Geometry check sheet. Reference: the model listing, model coordinates, mm. A direction names the side the tool comes from. Round coordinates to 2 decimals unless told otherwise and drop trailing zeros. Loops run counter-clockwise (first coordinate to the right, second up) from the corner with the lowest first, then second, coordinate; pieces in that order, holes last.
```python
from build123d import *

# Parameters (mm, degrees)
SKETCH1_W                   = 9
SKETCH1_H                   = 6
MAIN_BODY_EXT_DEPTH         = 8.3
EMISSION_PATH_EXT_DEPTH     = 9
SKETCH3_R                   = 1.25
EMISSION_AND_GRIN_CUT_DEPTH = 19.125672401
SKETCH4_R                   = 1
DRUM_LENS_CUT_DEPTH         = 7
SKETCH5_W                   = 9
SKETCH5_H                   = 7.3
FILTERSET_CUT1_DEPTH        = 1
FILTERSET_CUT2_DEPTH        = 4
SKETCH10_R                  = 2.5
EMISSION_LENS_CUT_DEPTH     = 8.5
SKETCH15_R                  = 0.795
MAGNETS_CUT_DEPTH           = 0.9
SCREW_HOLES_CUT_DEPTH       = 19.561788707
SCREW_HOLES_CUT_DEPTH_BACK  = 3
SKETCH18_R                  = 0.375
EXTERNAL_FILLET_1_R         = 1.5
CUT_EXTRUDE8_DEPTH          = 12.545128843
CUT_EXTRUDE8_DEPTH_BACK     = 4
SKETCH28_R                  = 1.5
CUT_EXTRUDE9_DEPTH          = 3
CUT_EXTRUDE10_DEPTH         = 0.7
SKETCH29_R                  = 0.375
CUT_EXTRUDE11_DEPTH         = 2.5
SKETCH32_W                  = 2
SKETCH32_H                  = 2.36
CUT_EXTRUDE14_DEPTH         = 0.7
CUT_EXTRUDE16_DEPTH         = 9
CUT_EXTRUDE17_REACH         = 12.329
SKETCH37_R                  = 2
CUT_EXTRUDE18_START         = -9
CUT_EXTRUDE18_DEPTH         = 9


with BuildPart() as part:
    # Sketch1 → Main Body Ext (new body)
    with BuildSketch(Plane(origin=(0, 0, 0), x_dir=(1, 0, 0), z_dir=(0, 1, 0))):
        Rectangle(SKETCH1_W, SKETCH1_H)
    extrude(amount=MAIN_BODY_EXT_DEPTH)

    # Sketch8 → Emission Path Ext (add)
    with BuildSketch(Plane(origin=(0, 8.3, 0), x_dir=(1, 0, 0), z_dir=(0, 1, 0))):
        Polygon((0.25, 3), (1.5, 1.75), (1.5, -3), (-4.5, -3), (-4.5, 3), align=None)
    extrude(amount=EMISSION_PATH_EXT_DEPTH)

    # Sketch3 → Emission and Grin Cut (cut, through all)
    with BuildSketch(Plane.XZ):
        with Locations(Location((-1.5, 0, 0), (0, 0, 270))):
            Circle(SKETCH3_R)
    extrude(amount=-EMISSION_AND_GRIN_CUT_DEPTH, mode=Mode.SUBTRACT)

    # Sketch4 → Drum Lens Cut (cut)
    with BuildSketch(Plane(origin=(4.5, 0, 0), x_dir=(0, 0, -1), z_dir=(1, 0, 0))):
        with Locations((0, 3)):
            Circle(SKETCH4_R)
    extrude(amount=-DRUM_LENS_CUT_DEPTH, mode=Mode.SUBTRACT)

    # Sketch5 → FilterSet Cut1 (cut)
    with BuildSketch(Plane.XY.offset(3)):
        with Locations((0, 4.65)):
            Rectangle(SKETCH5_W, SKETCH5_H)
    extrude(amount=-FILTERSET_CUT1_DEPTH, mode=Mode.SUBTRACT)

    # Sketch6 → FilterSet Cut2 (cut)
    with BuildSketch(Plane.XY.offset(2)):
        with BuildLine():
            Line((2.3, 4.5), (2.3, 1.8))
            ThreePointArc((2.3, 1.8), (2.7, 1.4), (2.3, 1))
            Line((2.3, 1), (1.1, 1))
            ThreePointArc((1.1, 1), (0.7, 1.4), (1.1, 1.8))
            Line((1.1, 1.8), (1.1, 4.5))
            ThreePointArc((1.1, 4.5), (1.7, 5.1), (2.3, 4.5))
        make_face()
        with BuildLine():
            Line((-3.9, 7.9), (-3.9, 7.5))
            ThreePointArc((-3.9, 7.5), (-3.782842712, 7.217157288), (-3.5, 7.1))
            Line((-3.5, 7.1), (0.5, 7.1))
            ThreePointArc((0.5, 7.1), (0.782842712, 7.217157288), (0.9, 7.5))
            Line((0.9, 7.5), (0.9, 7.9))
            ThreePointArc((0.9, 7.9), (0.782842712, 8.182842712), (0.5, 8.3))
            Line((0.5, 8.3), (-3.5, 8.3))
            ThreePointArc((-3.5, 8.3), (-3.782842712, 8.182842712), (-3.9, 7.9))
        make_face()
        with BuildLine():
            Line((0.39411255, 6.591168825), (-3.848528137, 2.348528137))
            ThreePointArc((-3.848528137, 2.348528137), (-3.848528137, 1.5), (-3, 1.5))
            Line((-3, 1.5), (1.242640687, 5.742640687))
            ThreePointArc((1.242640687, 5.742640687), (1.242640687, 6.591168825), (0.39411255, 6.591168825))
        make_face()
    extrude(amount=-FILTERSET_CUT2_DEPTH, mode=Mode.SUBTRACT)

    # Sketch10 → Emission Lens Cut (cut)
    with BuildSketch(Plane(origin=(0, 17.3, 0), x_dir=(1, 0, 0), z_dir=(0, 1, 0))):
        with Locations(Location((-1.5, 0, 0), (0, 0, 270))):
            Circle(SKETCH10_R)
    extrude(amount=-EMISSION_LENS_CUT_DEPTH, mode=Mode.SUBTRACT)

    # Sketch15 → Magnets Cut (cut)
    with BuildSketch(Plane.XZ):
        with Locations(Location((-3.25, -1.875, 0), (0, 0, 270))):
            Circle(SKETCH15_R)
        with Locations(Location((-3.25, 1.875, 0), (0, 0, 270))):
            Circle(SKETCH15_R)
        with Locations(Location((1.5, 0, 0), (0, 0, 270))):
            Circle(SKETCH15_R)
    extrude(amount=-MAGNETS_CUT_DEPTH, mode=Mode.SUBTRACT)

    # Sketch18 → Screw Holes Cut (cut, two sides: drawn at the far end of the back side and taken through both)
    with BuildSketch(Plane.XY.offset(2).offset(-SCREW_HOLES_CUT_DEPTH_BACK)):
        with Locations(Location((-3.5, 4, 0), (0, 0, 180))):
            Circle(SKETCH18_R)
        with Locations(Location((2.5, 6.5, 0), (0, 0, 180))):
            Circle(SKETCH18_R)
        with Locations((3.25, 1)):
            Circle(SKETCH18_R)
    extrude(amount=SCREW_HOLES_CUT_DEPTH + SCREW_HOLES_CUT_DEPTH_BACK, mode=Mode.SUBTRACT)

    # External Fillet 1
    # the kernel refuses this fillet: 1.5 mm, written as the material it takes off along each edge
    with BuildSketch(Plane(origin=(-4.5, -3.75, -3), x_dir=(1, 0, 0), z_dir=(0, 1, 0))) as external_fillet_1_piece_1:
        with BuildLine():
            CenterArc((EXTERNAL_FILLET_1_R, -EXTERNAL_FILLET_1_R), EXTERNAL_FILLET_1_R, 90, 90)
            Line((0, -EXTERNAL_FILLET_1_R), (0, 0))
            Line((0, 0), (EXTERNAL_FILLET_1_R, 0))
        make_face()
    extrude(amount=24.8, mode=Mode.SUBTRACT)
    with BuildSketch(Plane(origin=(1.5, 8.3, 3), x_dir=(0, 0, -1), z_dir=(0, 1, 0))) as external_fillet_1_piece_2:
        with BuildLine():
            CenterArc((EXTERNAL_FILLET_1_R, EXTERNAL_FILLET_1_R), EXTERNAL_FILLET_1_R, 180, 90)
            Line((0, EXTERNAL_FILLET_1_R), (0, 0))
            Line((0, 0), (EXTERNAL_FILLET_1_R, 0))
        make_face()
    extrude(amount=12.75, mode=Mode.SUBTRACT)

    # Sketch28 → Cut-Extrude8 (cut, two sides: drawn at the far end of the back side and taken through both)
    with BuildSketch(Plane(origin=(0, 7.1, 0), x_dir=(1, 0, 0), z_dir=(0, 1, 0)).offset(-CUT_EXTRUDE8_DEPTH_BACK)):
        with Locations(Location((-1.5, 0, 0), (0, 0, 180))):
            Circle(SKETCH28_R)
    extrude(amount=CUT_EXTRUDE8_DEPTH + CUT_EXTRUDE8_DEPTH_BACK, mode=Mode.SUBTRACT)

    # Sketch14 → Cut-Extrude9 (cut)
    with BuildSketch(Plane.XZ):
        Polygon((4.5, -3), (4.5, -2.006698359), (3.837798906, -3), align=None)
    extrude(amount=-CUT_EXTRUDE9_DEPTH, mode=Mode.SUBTRACT)

    # Sketch12 → Cut-Extrude10 (cut)
    with BuildSketch(Plane(origin=(4.5, 0, 0), x_dir=(0, 0, -1), z_dir=(1, 0, 0))):
        with BuildLine():
            Line((1.6, 5.94), (-1.6, 5.94))
            Line((-1.6, 5.94), (-2, 5.94))
            Line((-2, 5.94), (-2, 1.33))
            Line((-2, 1.33), (1.6, 1.33))
            ThreePointArc((1.6, 1.33), (1.882842712, 1.447157288), (2, 1.73))
            Line((2, 1.73), (2, 5.54))
            ThreePointArc((2, 5.54), (1.882842712, 5.822842712), (1.6, 5.94))
        make_face()
    extrude(amount=-CUT_EXTRUDE10_DEPTH, mode=Mode.SUBTRACT)

    # Sketch29 → Cut-Extrude11 (cut)
    with BuildSketch(Plane(origin=(4.5, 0, 0), x_dir=(0, 0, -1), z_dir=(1, 0, 0))):
        with Locations((2, 6.5)):
            Circle(SKETCH29_R)
    extrude(amount=-CUT_EXTRUDE11_DEPTH, mode=Mode.SUBTRACT)

    # Sketch32 → Cut-Extrude14 (cut)
    with BuildSketch(Plane(origin=(4.5, 0, 0), x_dir=(0, 0, -1), z_dir=(1, 0, 0))):
        with Locations((0, 7.12)):
            Rectangle(SKETCH32_W, SKETCH32_H)
    extrude(amount=-CUT_EXTRUDE14_DEPTH, mode=Mode.SUBTRACT)

    # Sketch33 → Cut-Revolve1 (revolve, cut)
    with BuildSketch(Plane.XY, mode=Mode.PRIVATE) as cut_revolve1_sk:
        with BuildLine():
            Line((3.8, 3), (2.3, 3))
            ThreePointArc((2.3, 3), (2.739339828, 4.060660172), (3.8, 4.5))
            Line((3.8, 4.5), (3.8, 3))
        make_face()
    revolve(cut_revolve1_sk.sketch.rotate(Axis((3.8, 3, 0), (-1, 0, 0)), 90), axis=Axis((3.8, 3, 0), (-1, 0, 0)), mode=Mode.SUBTRACT)

    # Sketch36 → Cut-Extrude16 (cut)
    with BuildSketch(Plane(origin=(0, 17.3, 0), x_dir=(1, 0, 0), z_dir=(0, 1, 0))):
        with BuildLine():
            Line((-4.5, -1.5), (-4.5, -3))
            Line((-4.5, -3), (-3, -3))
            ThreePointArc((-3, -3), (-4.060660172, -2.560660172), (-4.5, -1.5))
        make_face()
    extrude(amount=-CUT_EXTRUDE16_DEPTH, mode=Mode.SUBTRACT)

    # Sketch37 → Cut-Extrude17 (cut, up to next)
    with BuildSketch(Plane(origin=(0, 8.8, 0), x_dir=(1, 0, 0), z_dir=(0, 1, 0)), mode=Mode.PRIVATE) as cut_extrude17_sk1:
        with Locations(Location((-1.5, 0, 0), (0, 0, 180))):
            Circle(SKETCH37_R)
    cut_extrude17_tool1 = extrude(cut_extrude17_sk1.sketch, amount=-CUT_EXTRUDE17_REACH, mode=Mode.PRIVATE) & part.part
    add(cut_extrude17_tool1.solids().sort_by_distance((-1.5, 8.8, 0))[0], mode=Mode.SUBTRACT)

    # Sketch38 → Cut-Extrude18 (cut)
    with BuildSketch(Plane(origin=(0, 17.3, 0), x_dir=(1, 0, 0), z_dir=(0, 1, 0)).offset(CUT_EXTRUDE18_START)):
        with BuildLine():
            Line((-3, 3), (0.25, 3))
            Line((0.25, 3), (1.5, 1.75))
            Line((1.5, 1.75), (1.5, -1.5))
            ThreePointArc((1.5, -1.5), (1.060660172, -2.560660172), (0, -3))
            Line((0, -3), (-3, -3))
            ThreePointArc((-3, -3), (-4.060660172, -2.560660172), (-4.5, -1.5))
            Line((-4.5, -1.5), (-4.5, 1.5))
            ThreePointArc((-4.5, 1.5), (-4.060660172, 2.560660172), (-3, 3))
        make_face()
        with BuildLine():
            Line((-4.375, -1.5), (-4.375, 1.5))
            ThreePointArc((-4.375, 1.5), (-3.940482173, 2.440482173), (-3, 2.875))
            Line((-3, 2.875), (0.25, 2.875))
            Line((0.25, 2.875), (1.375, 1.75))
            Line((1.375, 1.75), (1.375, -1.5))
            ThreePointArc((1.375, -1.5), (0.972271824, -2.472271824), (0, -2.875))
            Line((0, -2.875), (-3, -2.875))
            ThreePointArc((-3, -2.875), (-3.972271824, -2.472271824), (-4.375, -1.5))
        make_face(mode=Mode.SUBTRACT)
    extrude(amount=CUT_EXTRUDE18_DEPTH, mode=Mode.SUBTRACT)


solid = part.part
```
1) Access from +Z, -Z, +X, -X, +Y, -Y to the whole of each face (thin tool, end or side, straight path). Record for faces 1 (the face through (0.805, 12.737, -2.32)), 2 (the face through (-3.1, 8.3, -1.5)), 3 (the face through (-1, 13, -2.875)).
Report:
face 1: -Z, +X, +Y
face 2: +Z
face 3: -Z, +X, -X, +Y
2) Gauge pin test, flat ends, axial feed: pin 1 (1 mm diameter, centred on y = 10.5, z = -2, fed in from -X) (3 decimals); pin 2 (2 mm diameter, centred on x = 3.5, z = -2, fed in from +Y); pin 3 (1.3 mm diameter, centred on x = -2, y = 8, fed in from +Z) (3 decimals). Record the tip position at first contact, or that the pin passes through.
Report:
pin 1: stops at x = -4.375
pin 2: stops at y = 8.3
pin 3: stops at z = 2.875
3) Sectioned sample at C-C, the plane z = -0.35. State how many separate pieces and enclosed holes the cut face has, then the cut area to 3 significant figures.
Report:
separate pieces: 3
enclosed holes: 3
area: 35.1 mm2
4) Mould release check, pull along Y, two halves, no side actions. Record for faces 4 (the face through (-1, 4, -2)), 5 (the face through (-4, 17.3, -1)), 6 (the face through (0.1, 0.5, 3)): +Y half, -Y half, draft (parallel to the pull), parting line (faces both ways), or undercut.
Report:
face 4: undercut
face 5: +Y half
face 6: draft
5) Scan lines: line 1 along Y through (x, z) = (-3.5, 1.3) (3 decimals); line 2 along Z through (x, y) = (-1.5, 5.15); line 3 along Y through (x, z) = (0, -0.75). Record each from-to range of solid material in increasing order.
Report:
line 1: y = 0.9 to 1.329, 2.697 to 3.625, 4.375 to 7.1, 8.3 to 8.8
line 2: z = -3 to -1.5, 1.5 to 2
line 3: y = 0 to 2.34, 3.66 to 4.5, 6.2 to 7.1
6) Sectioned sample at B-B, the plane x = 3.25. Record the cut outline in (y, z) (3 decimals).
Report:
outline: (0, -3) - (8.3, -3) - (8.3, 2) - (1.375, 2) - (1.375, -1) - (0.625, -1) - (0.625, 3) - (0, 3) - close; hole circle Ø2.791 at (3, 0); hole circle Ø0.75 at (6.5, -2)
7) Sectioned sample at A-A, the plane y = 14. Record the cut outline in (x, z) (3 decimals).
Report:
outline: (-4.375, -1.5) arc R1.5 ccw to (-3, -2.875) - (0.25, -2.875) - (1.375, -1.75) - (1.375, 1.5) arc R1.375 ccw to (0, 2.875) - (-3, 2.875) arc R1.375 ccw to (-4.375, 1.5) - close; hole circle Ø5 at (-1.5, 0)
